Source: CAD feature listing. Evaluate the final solid. Frame: model axes, mm. Give positions to 0.01 mm unless a question says otherwise; leave off trailing zeros. Write each loop counter-clockwise with the first axis right and the second up, starting at its lowest first coordinate (ties: lowest second). Pieces come first, ordered by that corner, then holes. Notation, with made-up numbers: M 64,50.5 L 115,50.5 A30 cw 115,87.5 Z; hole C -28.75,-25.75 d2. An arc over 180 degrees is marked long. Answer as a JSON object with one key per item and string values. Group by question number.
Autodesk Inventor part; units mm, degrees
ref_plane "YZ Plane" through (0, 0, 0) normal (1, 0, 0) x (0, 1, 0)
ref_plane "XZ Plane" through (0, 0, 0) normal (0, 1, 0) x (-1, 0, 0)
ref_plane "XY Plane" through (0, 0, 0) normal (0, 0, 1) x (1, 0, 0)
sketch "Sketch1" plane through (0, 0, 0) normal (0, 0, 1) x (1, 0, 0)
  line L0 (-75, -75) -> (75, -75)
  line L1 (75, -75) -> (75, 75)
  line L2 (75, 75) -> (-75, 75)
  line L3 (-75, 75) -> (-75, -75)
  line L4 (-75, -75) -> (75, 75) construction
  line L5 (75, -75) -> (-75, 75) construction
  circle A0 centre (0, 0) radius 20
  point P0 (25, 25)
  dimension "d0" = 150
  dimension "d1" = 150
  dimension "d2" = 40
  dimension "d5" = 25
extrude "Extrusion1" add sketch "Sketch1" along normal blind 6
hole "Hole1" at (25, 25, 0) direction (0, 0, 1) diameter 3 end through all
pattern_circular "Circular Pattern1" count 6 over 360 about axis through (0, 0, 0) along (0, 0, 1) of "Hole1"
properties part number "base_plate" material "Plywood, Finish"
(1) Section A-A, the plane y = 0. Return loops of the section in (x, z), plus the area to 3 significant figures.
(2) Section C-C, the plane z = 2.65. Return loops of the section in (x, y).
(3) Contact query for a flat-ended pin moving along its axis: pin 1 Ø2.5 at (x, y) = (25, 25) entering from -Z. Output: stop coordinate, or through.
(4) Pull-direction query (Y, two-part tool) for faces 1 (the flat face through (1, 75, 3)), 2 (the cylindrical face through (-4.336, 19.524, 2.958)), 3 (the flat face through (-1, -75, 3)), 4 (the flat face through (75, -1, 3)); classes: pulls with the +Y half, pulls with the -Y half, needs draft (parallel to the pull), parting line crosses it, or undercut.
(5) Ray query, L1, parallel to X at y = 25, z = 2.9; L2, parallel to Y at x = 1, z = 5.45; L3, parallel to X at y = -0.5, z = 3.2. Return the intervals inside material, ascending. Write a range as [from, to].
Reported:
{
 "1": {"outline": "M -75,0 L -20,0 L -20,6 L -75,6 Z; M 20,0 L 75,0 L 75,6 L 20,6 Z", "area": "660 mm2"},
 "2": {"outline": "M -75,-75 L 75,-75 L 75,75 L -75,75 Z; hole C -34.15,9.15 d3; hole C -25,-25 d3; hole C 0,0 d40; hole C -9.15,34.15 d3; hole C 9.15,-34.15 d3; hole C 25,25 d3; hole C 34.15,-9.15 d3"},
 "3": {"pin 1": "passes through"},
 "4": {"face 1": "pulls with the +Y half", "face 2": "undercut", "face 3": "pulls with the -Y half", "face 4": "needs draft"},
 "5": {"L1": "x = [-75, 23.5], [26.5, 75]", "L2": "y = [-75, -19.97], [19.97, 75]", "L3": "x = [-75, -19.99], [19.99, 75]"}
}
